Geometry check sheet. Reference: the model listing, model coordinates, mm. Face numbers are marked on the shaded views. A direction names the side the tool comes from. Round coordinates to 2 decimals unless told otherwise and drop trailing zeros. Loops run counter-clockwise (first coordinate to the right, second up) from the corner with the lowest first, then second, coordinate; pieces in that order, holes last. Notation, with made-up numbers: (47, 13) -> (63, 13) arc R17 cw to (63, 34) -> close; hole circle Ø7 at (-5, 48). An arc over 180 degrees is marked (long way). Use one line per item in the form item = value.
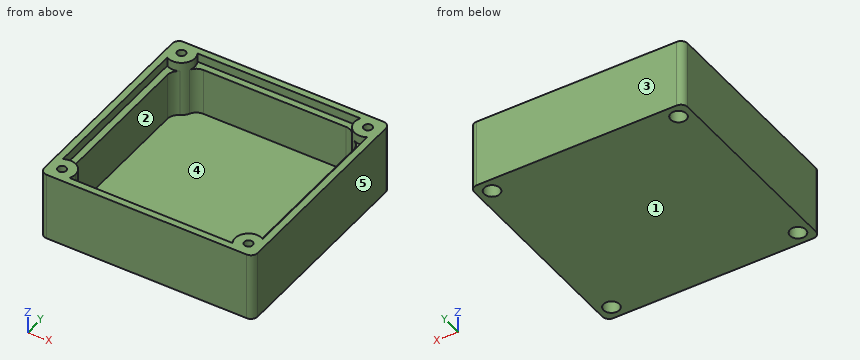
from build123d import *

# Parameters (mm, degrees)
F0_W        = 95
F0_H        = 95
F1_DEPTH    = 30.5
F3_DEPTH    = 25
F4_R        = 1.9
F5_DEPTH    = 30.501
F6_R        = 3
F7_W        = 72.6076951546
F7_H        = 3
F7_W_2      = 3
F7_H_2      = 72.6076951546
F8_DEPTH    = 21
F9_T1_DEPTH = 21
F10_R       = 3.5
F11_DEPTH   = 15.5


# Not quite as in the source:
# - a fillet or chamfer that OpenCascade refuses, or shapes differently, is made with other operations: its cross-section is extruded or revolved along the edge and cut away or added


with BuildPart() as f1:
    # F0 (on Top) → F1 (new body)
    with BuildSketch(Plane.XY):
        Rectangle(F0_W, F0_H)
    extrude(amount=F1_DEPTH)

    # F2 (on face) → F3 (cut)
    with BuildSketch(Plane.XY.offset(30.5)):
        with BuildLine():
            Line((36.3038475773, 44.5), (-36.3038475773, 44.5))
            ThreePointArc((-36.3038475773, 44.5), (-35.7044450423, 43.0529142706), (-35.5, 41.5))
            ThreePointArc((-35.5, 41.5), (-38.5, 36.3038475773), (-44.5, 36.3038475773))
            Line((-44.5, 36.3038475773), (-44.5, -36.3038475773))
            ThreePointArc((-44.5, -36.3038475773), (-38.5, -36.3038475773), (-35.5, -41.5))
            ThreePointArc((-35.5, -41.5), (-35.7044450423, -43.0529142706), (-36.3038475773, -44.5))
            Line((-36.3038475773, -44.5), (36.3038475773, -44.5))
            ThreePointArc((36.3038475773, -44.5), (37.2573593129, -37.2573593129), (44.5, -36.3038475773))
            Line((44.5, -36.3038475773), (44.5, 36.3038475773))
            ThreePointArc((44.5, 36.3038475773), (37.2573593129, 37.2573593129), (36.3038475773, 44.5))
        make_face()
    extrude(amount=-F3_DEPTH, mode=Mode.SUBTRACT)

    # F4 (on face) → F5 (cut, through all)
    with BuildSketch(Plane.XY.offset(30.5)):
        with Locations((-41.5, 41.5)):
            Circle(F4_R)
        with Locations((41.5, 41.5)):
            Circle(F4_R)
        with Locations((-41.5, -41.5)):
            Circle(F4_R)
        with Locations((41.5, -41.5)):
            Circle(F4_R)
    extrude(amount=-F5_DEPTH, mode=Mode.SUBTRACT)

    # F6
    f6_edges = [f1.edges().sort_by_distance(p)[0] for p in [
        (-47.5, 47.5, 15.25),
        (47.5, 47.5, 15.25),
        (-47.5, -47.5, 15.25),
        (47.5, -47.5, 15.25),
    ]]
    fillet(f6_edges, radius=F6_R)

    # F7 (on face) → F8 (join)
    with BuildSketch(Plane.XY.offset(5.5)):
        with Locations((0, 43)):
            Rectangle(F7_W, F7_H)
        with Locations((-43, 0)):
            Rectangle(F7_W_2, F7_H_2)
        with Locations((0, -43)):
            Rectangle(F7_W, F7_H)
        with Locations((43, 0)):
            Rectangle(F7_W_2, F7_H_2)
    extrude(amount=F8_DEPTH)

    # F9: fillet of radius 5 on 8 edges, made by hand

    # F9_s2 → F9_t1 (join)
    with BuildSketch(Plane.XY.offset(5.5)):
        with BuildLine():
            ThreePointArc((-36.155658743, 38.7727272727), (-34.3132058682, 40.7640143271), (-31.7020410289, 41.5))
            Line((-31.7020410289, 41.5), (-35.5, 41.5))
            ThreePointArc((-35.5, 41.5), (-35.6662170274, 40.0975107027), (-36.155658743, 38.7727272727))
        make_face()
        with BuildLine():
            ThreePointArc((-38.7727272727, 36.155658743), (-40.7640143271, 34.3132058682), (-41.5, 31.7020410289))
            Line((-41.5, 31.7020410289), (-41.5, 35.5))
            ThreePointArc((-41.5, 35.5), (-40.0975107027, 35.6662170274), (-38.7727272727, 36.155658743))
        make_face()
        with BuildLine():
            ThreePointArc((36.155658743, 38.7727272727), (34.3132058682, 40.7640143271), (31.7020410289, 41.5))
            Line((31.7020410289, 41.5), (35.5, 41.5))
            ThreePointArc((35.5, 41.5), (35.6662170274, 40.0975107027), (36.155658743, 38.7727272727))
        make_face()
        with BuildLine():
            ThreePointArc((38.7727272727, 36.155658743), (40.7640143271, 34.3132058682), (41.5, 31.7020410289))
            Line((41.5, 31.7020410289), (41.5, 35.5))
            ThreePointArc((41.5, 35.5), (40.0975107027, 35.6662170274), (38.7727272727, 36.155658743))
        make_face()
        with BuildLine():
            ThreePointArc((38.7727272727, -36.155658743), (40.7640143271, -34.3132058682), (41.5, -31.7020410289))
            Line((41.5, -31.7020410289), (41.5, -35.5))
            ThreePointArc((41.5, -35.5), (40.0975107027, -35.6662170274), (38.7727272727, -36.155658743))
        make_face()
        with BuildLine():
            ThreePointArc((36.155658743, -38.7727272727), (34.3132058682, -40.7640143271), (31.7020410289, -41.5))
            Line((31.7020410289, -41.5), (35.5, -41.5))
            ThreePointArc((35.5, -41.5), (35.6662170274, -40.0975107027), (36.155658743, -38.7727272727))
        make_face()
        with BuildLine():
            ThreePointArc((-38.7727272727, -36.155658743), (-40.7640143271, -34.3132058682), (-41.5, -31.7020410289))
            Line((-41.5, -31.7020410289), (-41.5, -35.5))
            ThreePointArc((-41.5, -35.5), (-40.0975107027, -35.6662170274), (-38.7727272727, -36.155658743))
        make_face()
        with BuildLine():
            ThreePointArc((-36.155658743, -38.7727272727), (-34.3132058682, -40.7640143271), (-31.7020410289, -41.5))
            Line((-31.7020410289, -41.5), (-35.5, -41.5))
            ThreePointArc((-35.5, -41.5), (-35.6662170274, -40.0975107027), (-36.155658743, -38.7727272727))
        make_face()
    extrude(amount=F9_T1_DEPTH)

    # F10 (on face) → F11 (cut)
    with BuildSketch(Plane(origin=(0, 0, 0), x_dir=(1, 0, 0), z_dir=(0, 0, -1))):
        with Locations((-41.5, 41.5)):
            Circle(F10_R)
        with Locations((41.5, 41.5)):
            Circle(F10_R)
        with Locations((-41.5, -41.5)):
            Circle(F10_R)
        with Locations((41.5, -41.5)):
            Circle(F10_R)
    extrude(amount=-F11_DEPTH, mode=Mode.SUBTRACT)


solid = f1.part
1. Mould release check, pull along X, two halves, no side actions. Record for the marked faces 3, 4 and 5: released by +X, released by -X, zero draft, split by the parting line, or undercut.
Return value:
face_3 = zero draft
face_4 = undercut
face_5 = released by +X
2. Tool access check on the marked faces 1 and 2. Record the directions out of +Z, -Z, +X, -X, +Y, -Y that give a thin tool (end or side, any length) a straight path to the whole face; none if there is none.
Return value:
face_1 = -Z, +X, -X, +Y, -Y
face_2 = +Z
3. Section check B-B (x = -13). Record the boundary of the cut face in (y, z).
Return value:
outline = (-47.5, 0) -> (47.5, 0) -> (47.5, 30.5) -> (44.5, 30.5) -> (44.5, 26.5) -> (41.5, 26.5) -> (41.5, 5.5) -> (-41.5, 5.5) -> (-41.5, 26.5) -> (-44.5, 26.5) -> (-44.5, 30.5) -> (-47.5, 30.5) -> close
4. Section check A-A (z = 24). Record the boundary of the cut face in (x, y).
Return value:
outline = (-47.5, -44.5) arc R3 ccw to (-44.5, -47.5) -> (44.5, -47.5) arc R3 ccw to (47.5, -44.5) -> (47.5, 44.5) arc R3 ccw to (44.5, 47.5) -> (-44.5, 47.5) arc R3 ccw to (-47.5, 44.5) -> close; hole circle Ø3.8 at (-41.5, -41.5); hole circle Ø3.8 at (-41.5, 41.5); hole (-41.5, -31.7) arc R5 ccw to (-38.77, -36.16) arc R6 cw to (-36.16, -38.77) arc R5 ccw to (-31.7, -41.5) -> (31.7, -41.5) arc R5 ccw to (36.16, -38.77) arc R6 cw to (38.77, -36.16) arc R5 ccw to (41.5, -31.7) -> (41.5, 31.7) arc R5 ccw to (38.77, 36.16) arc R6 cw to (36.16, 38.77) arc R5 ccw to (31.7, 41.5) -> (-31.7, 41.5) arc R5 ccw to (-36.16, 38.77) arc R6 cw to (-38.77, 36.16) arc R5 ccw to (-41.5, 31.7) -> close; hole circle Ø3.8 at (41.5, -41.5); hole circle Ø3.8 at (41.5, 41.5)
5. Gauge pin test, flat ends, axial feed: pin 1 (4.5 mm diameter, centred on x = 11, y = -42, fed in from +Z); pin 2 (4 mm diameter, centred on x = -41.5, y = 41.5, fed in from -Z); pin 3 (8 mm diameter, centred on x = -11.5, y = -23, fed in from +Z); pin 4 (2 mm diameter, centred on x = -42, y = -41.5, fed in from -Z). Record the tip position at first contact, or that the pin passes through.
Return value:
pin_1 = 26.5
pin_2 = 15.5
pin_3 = 5.5
pin_4 = through
6. Material ranges on line 1 along X through (y, z) = (-41.5, 4.5); line 2 along X through (y, z) = (9, 25); line 3 along Y through (x, z) = (-41, 21), recorded low to high.
Return value:
line_1 = -47.5 to -45, -38 to 38, 45 to 47.5
line_2 = -47.5 to -41.5, 41.5 to 47.5
line_3 = -47.5 to -43.33, -39.67 to -33.88, 33.88 to 39.67, 43.33 to 47.5
